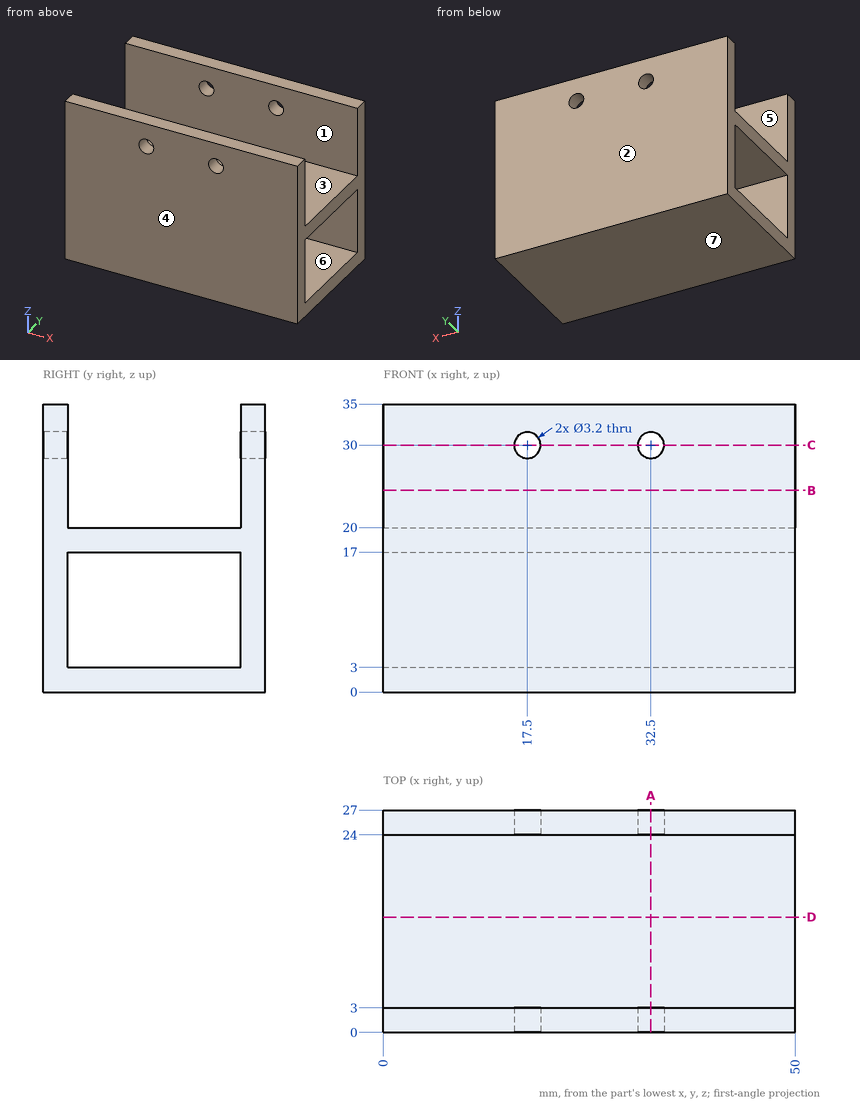
Input: dimensioned drawing with shaded views. Units: mm. Origin: part minimum x, y, z. A direction names the side the tool comes from. Give positions to 0.01 mm unless a question says otherwise; leave off trailing zeros. Order: outer loops, then holes, each group sorted by start corner. A loop starts at its lowest first (then second) coordinate and runs counter-clockwise, first axis right, second up. Notation, with made-up numbers: (68.5, -40) -> (112.5, -40) arc R13 ccw to (112.5, -35) -> close; hole circle Ø7 at (63.25, -7). An arc over 180 degrees is marked (long way). Write item = value, one per line.
Item 1: Section query A-A (x = 32.5). Output: boundary loops of the cut face in (y, z), then the cut area to 3 significant figures.
Check result:
outline = (0, 0) -> (27, 0) -> (27, 28.4) -> (24, 28.4) -> (24, 20) -> (3, 20) -> (3, 28.4) -> (0, 28.4) -> close; (0, 31.6) -> (3, 31.6) -> (3, 35) -> (0, 35) -> close; (24, 31.6) -> (27, 31.6) -> (27, 35) -> (24, 35) -> close; hole (3, 3) -> (24, 3) -> (24, 17) -> (3, 17) -> close
area = 317 mm²
Item 2: Section query C-C (z = 30). Output: boundary loops of the cut face in (x, y).
Check result:
outline = (0, 0) -> (15.9, 0) -> (15.9, 3) -> (0, 3) -> close; (0, 24) -> (15.9, 24) -> (15.9, 27) -> (0, 27) -> close; (19.1, 0) -> (30.9, 0) -> (30.9, 3) -> (19.1, 3) -> close; (19.1, 24) -> (30.9, 24) -> (30.9, 27) -> (19.1, 27) -> close; (34.1, 0) -> (50, 0) -> (50, 3) -> (34.1, 3) -> close; (34.1, 24) -> (50, 24) -> (50, 27) -> (34.1, 27) -> close
Item 3: Mould query, pull axis Y, two halves, no side actions, for the marked faces 1, 2, 3 and 4. Classes: +Y half, -Y half, draft (parallel to the pull), parting line (faces both ways), or undercut.
Check result:
face_1 = undercut
face_2 = +Y half
face_3 = undercut
face_4 = -Y half
Item 4: Contact query for a flat-ended pin moving along its axis: pin 1 (4 mm diameter, centred on x = 26, y = 8.5, fed in from +Z). Output: stop coordinate, or through.
Check result:
pin_1 = 20
Item 5: Ray query, probe 1 along X at (y, z) = (25, 30); probe 2 along Y at (x, z) = (43, 22.5); probe 3 along Z at (x, y) = (44, 9.5). Return the intervals inside material, ascending.
Check result:
probe_1 = 0 to 15.9, 19.1 to 30.9, 34.1 to 50
probe_2 = 0 to 3, 24 to 27
probe_3 = 0 to 3, 17 to 20
Item 6: Set-up query: the marked faces 5, 6 and 7. Return all of +Z, -Z, +X, -X, +Y, -Y with unobstructed straight access to the full face (end or side cutting, diameter ignored); none if empty.
Check result:
face_5 = +Z, +X, -X
face_6 = +X, -X
face_7 = -Z, +X, -X, +Y, -Y
Item 7: Section query D-D (y = 14). Output: boundary loops of the cut face in (x, z), then the cut area to 3 significant figures.
Check result:
outline = (0, 0) -> (50, 0) -> (50, 3) -> (0, 3) -> close; (0, 17) -> (50, 17) -> (50, 20) -> (0, 20) -> close
area = 300 mm²
Item 8: Section query B-B (z = 24.5). Output: boundary loops of the cut face in (x, y).
Check result:
outline = (0, 0) -> (50, 0) -> (50, 3) -> (0, 3) -> close; (0, 24) -> (50, 24) -> (50, 27) -> (0, 27) -> close
